```python
from build123d import *

# Parameters (mm, degrees)
F1_DEPTH = 9.525


# Not quite as in the source:
# - a length typed as a fraction of an inch, garbled in the dataset ("3 / 203.2 mm" for 3/8 in), is restored


with BuildPart() as f1:
    # F0 (on Front) → F1 (new body)
    with BuildSketch(Plane.XZ):
        with BuildLine():
            ThreePointArc((0, 152.4), (-107.7630734528, -107.7630734528), (152.4, 0))
            ThreePointArc((152.4, 0), (107.7630734528, 107.7630734528), (0, 152.4))
        make_face()
        with BuildLine():
            Line((-12.7, 139.7), (0, 139.7))
            Line((0, 139.7), (12.7, 139.7))
            ThreePointArc((12.7, 139.7), (14.9450640303, 138.7700640303), (15.875, 136.525))
            ThreePointArc((15.875, 136.525), (14.9450640303, 134.2799359697), (12.7, 133.35))
            Line((12.7, 133.35), (0, 133.35))
            Line((0, 133.35), (-12.7, 133.35))
            ThreePointArc((-12.7, 133.35), (-15.875, 136.525), (-12.7, 139.7))
        make_face(mode=Mode.SUBTRACT)
    extrude(amount=F1_DEPTH)


solid = f1.part
```
CAD build for the part. Positions are in the model's coordinates, mm. A direction names the side the tool comes from. Coordinates: 2 decimals unless noted, no trailing zeros. Write each loop counter-clockwise with the first axis right and the second up, starting at its lowest first coordinate (ties: lowest second). Pieces come first, ordered by that corner, then holes. Notation, with made-up numbers: (-35.5, -37.5) -> (-24.5, -37.5) arc R19 cw to (-24.5, -20.5) -> close; hole circle Ø10 at (40, 59.25). An arc over 180 degrees is marked (long way). Return JSON: item names as keys, results as strings. Group by question number.
Q1. Cut at B-B, the plane y = -8. Give the cut face in (x, z) (3 decimals).
Q2. Cut at C-C, the plane z = 59.5. Give the cut face in (x, y) (3 decimals).
Q3. Drill centre lines: line 1 (Z direction, x = 3, y = -8); line 2 (X direction, y = -3.5, z = -0.5); line 3 (Z direction, x = 6.5, y = -1.25). Where is each one in solid material? Low to high.
Q4. Cut at A-A, the plane x = 0. Give the cut face in (y, z) (3 decimals), then the cut area to 3 significant figures.
Q5. Which spindle directions (+Z, -Z, +X, -X, +Y, -Y) get a long thin tool onto all of the face, cutting with end or side? Do faces 1 (the face through (-2, 0, 2)), 2 (the face through (0, -5, 139.7)). Say none if no direction does.
Q6. Cut at D-D, the plane x = 37. Give the cut face in (y, z) (3 decimals), then the cut area to 3 significant figures.
Q7. Pull direction Z, two halves, no side cores. Call faces 3 (the face through (-120.94, -4.7, -92.73)), 4 (the face through (0, -5, 133.35)), 5 (the face through (-2, -9.525, 2)): released by +Z, released by -Z, zero draft, split by the parting line, or undercut.
Returned:
{
 "1": {"outline": "circle Ø304.8 at (0, 0); hole (-12.7, 133.35) -> (12.7, 133.35) arc R3.175 ccw to (12.7, 139.7) -> (-12.7, 139.7) arc R3.175 ccw to start"},
 "2": {"outline": "(-140.305, -9.525) -> (140.305, -9.525) -> (140.305, 0) -> (-140.305, 0) -> close"},
 "3": {"line 1": "z = -152.37 to 133.35, 139.7 to 152.37", "line 2": "x = -152.4 to 152.4", "line 3": "z = -152.26 to 133.35, 139.7 to 152.26"},
 "4": {"outline": "(-9.525, -152.4) -> (0, -152.4) -> (0, 133.35) -> (-9.525, 133.35) -> close; (-9.525, 139.7) -> (0, 139.7) -> (0, 152.4) -> (-9.525, 152.4) -> close", "area": "2,840 mm2"},
 "5": {"face 1": "+Z, -Z, +X, -X, +Y", "face 2": "+Y, -Y"},
 "6": {"outline": "(-9.525, -147.84) -> (0, -147.84) -> (0, 147.84) -> (-9.525, 147.84) -> close", "area": "2,820 mm2"},
 "7": {"face 3": "split by the parting line", "face 4": "undercut", "face 5": "zero draft"}
}
